Autodesk Inventor part; units mm, degrees
ref_plane "YZ Plane" through (0, 0, 0) normal (1, 0, 0) x (0, 1, 0)
ref_plane "XZ Plane" through (0, 0, 0) normal (0, 1, 0) x (-1, 0, 0)
ref_plane "XY Plane" through (0, 0, 0) normal (0, 0, 1) x (1, 0, 0)
sketch "Sketch1" plane through (0, 0, 0) normal (0, 1, 0) x (-1, 0, 0)
  line L0 (0, 0) -> (25, 0)
  line L1 (25, 0) -> (25, -28)
  line L2 (25, -28) -> (0, -28)
  line L3 (0, -28) -> (0, 0)
  dimension "d0" = 25
  dimension "d1" = 28
extrude "Extrusion1" add sketch "Sketch1" along normal blind 15
sketch "Sketch2" plane through (0, 15, 0) normal (0, 1, 0) x (1, 0, 0)
  point P0 (0, 0)
shell "Shell1" thickness 2 removed faces 1 at (-8.3333, 15, -9.3333)
sketch "Sketch3" plane through (0, 0, 0) normal (1, 0, 0) x (0, 0, -1)
  point P0 (0, 0)
sketch "Sketch4" plane through (0, 0, 0) normal (1, 0, 0) x (0, 0, -1)
  line L0 (0, 0) -> (0, 15)
  line L1 (0, 15) -> (0, 0)
  line L2 (0, 0) -> (-20, 0)
  line L3 (-20, 0) -> (-20, 2)
  arc A0 (-19, 3) -> (-20, 2) centre (-19, 2) ccw
  arc A1 (-19, 3) -> (-9.089, 9.2596) centre (-19, 13.976) ccw
  line L4 (28, 15) -> (0, 15)
  arc A2 (0, 15) -> (-9.089, 9.2596) centre (0, 4.9343) ccw
  line L5 (0, 15) -> (28, 15)
  dimension "d5" = 20
  dimension "d6" = 2
  dimension "d7" = 1
extrude "Extrusion2" add sketch "Sketch4" against normal blind 25
sketch "Sketch5" plane through (0, 0, -28) normal (0, 0, -1) x (-1, 0, 0)
  circle A0 centre (12.5, 13) radius 1.25
  line L0 (11.25, 13) -> (11.25, 15)
  line L1 (0, 15) -> (25, 15)
  line L2 (11.25, 15) -> (13.75, 15)
  line L3 (13.75, 15) -> (13.75, 13)
  point P0 (0, 0)
  dimension "d10" = 2.5
sketch "Sketch6" plane through (0, 0, -28) normal (0, 0, -1) x (-1, 0, 0)
  point P0 (0, 0)
extrude "Extrusion3" cut sketch "Sketch5" against normal up to next
sketch "Sketch7" plane through (-23, 2, -2) normal (0, 1, 0) x (1, 0, 0)
  point P0 (23, -2)
sketch "Sketch8" plane through (0, 15, 0) normal (0, 1, 0) x (1, 0, 0)
  line L0 (-2, 0) -> (-23, 0)
  line L1 (-23, 0) -> (-23, -20)
  line L2 (-23, -20) -> (-2, -20)
  line L3 (-2, -20) -> (-2, 0)
  line L4 (-12.5, 0) -> (-7.5, 0)
  line L5 (-7.5, 0) -> (-7.5, 2)
  line L6 (-7.5, 2) -> (-12.5, 2)
  line L7 (-12.5, 2) -> (-12.5, 0)
  line L8 (-12.5, 0) -> (-17.5, 0)
  line L9 (-17.5, 0) -> (-17.5, 2)
  line L10 (-17.5, 2) -> (-12.5, 2)
  line L11 (-12.5, 2) -> (-12.5, 0)
  point P0 (0, 0)
  dimension "d13" = 21
  dimension "d14" = 20
  dimension "d15" = 5
  dimension "d16" = 2
  dimension "d17" = 5
  dimension "d18" = 2
extrude "Extrusion4" cut sketch "Sketch8" against normal up to surface (13 mm away) contours L3 L2 L1 L0
extrude "Extrusion5" cut sketch "Sketch8" against normal blind 10 contours L0 L7 L6 L5 | L0 L9 L10 L7
sketch "Sketch9" plane through (-23, 2, -2) normal (0, 1, 0) x (1, 0, 0)
  line L0 (5.5, 0) -> (15.5, 0)
  line L1 (5.5, 0) -> (15.5, 0)
  line L2 (15.5, 0) -> (15.5, 10)
  line L3 (15.5, 10) -> (5.5, 10)
  line L4 (5.5, 10) -> (5.5, 0)
  point P0 (23, -2)
  dimension "d23" = 10
  dimension "d24" = 10
extrude "Extrusion6" add sketch "Sketch9" along normal up to surface (3 mm away)
properties part number "Holster"
Design review of the part built by this model. Coordinates are the model's own, in mm. A direction names the side the tool comes from. Give positions to 0.01 mm unless a question says otherwise; leave off trailing zeros. Order: outer loops, then holes, each group sorted by start corner. A loop starts at its lowest first (then second) coordinate and runs counter-clockwise, first axis right, second up. Notation, with made-up numbers: (40, 4.25) -> (76, 4.25) arc R20 ccw to (76, 35.25) -> close; hole circle Ø10 at (12.5, 56). An arc over 180 degrees is marked (long way). Write item = value, one per line. Start each with the question number.
(1) To check wall thickness, follow line 1 along X through (y, z) = (14, -13); line 2 along Z through (x, y) = (-22.25, 2.75); line 3 along X through (y, z) = (13.5, -0.5). State the ranges of each line that lie inside material, in increasing order.
(2) For pin 1 (4 mm diameter, centred on x = -9, y = 8, fed in from +Z); pin 2 (1.5 mm diameter, centred on x = -17, z = -22, fed in from +Y), all flat-tipped, find the tip position at first contact; note any pin that passes through.
(3) We need section C-C on x = -18. Write out the cut boundary in (y, z), plus the area to 3 significant figures.
(4) For faces 1 (the face through (-11.25, 14, -27)), 2 (the face through (-13, 5, -6)), 3 (the face through (-23, 8, -14)), 4 (the face through (-23.986, 13.487, 5.308)), 5 (the face through (-12, 1, 20)), list the 3-axis set-ups (+Z, -Z, +X, -X, +Y, -Y) from which the entire face can be reached by the end or side of a thin tool; tool diameter is ignored.
(5) We need section B-B on z = -7. Write out the cut boundary in (x, y), plus the area to 3 significant figures.
(6) We need section D-D on z = -23.5. Write out the cut boundary in (x, y).
(7) Mouldability with a two-part tool opening along X and no side actions: class faces 6 (the face through (-20, 8, -2)), 7 (the face through (-25, 7, -9)), 8 (the face through (0, 7, -10)) as +X half, -X half, draft (parallel to the pull), parting line (faces both ways), or undercut.
(8) We need section A-A on x = -8.25. Write out the cut boundary in (y, z), plus the area to 3 significant figures.
Numbers:
q1.line_1 = -25 to -23, -2 to 0
q1.line_2 = -28 to -26, -2 to 0
q1.line_3 = -25 to -17.5, -7.5 to 0
q2.pin_1 = 0
q2.pin_2 = 2
q3.outline = (0, -28) -> (15, -28) -> (15, -26) -> (2, -26) -> (2, -2) -> (15, -2) -> (15, 0) -> (2, 0) -> (2, 20) -> (0, 20) -> close
q3.area = 148 mm^2
q4.face_1 = +Z, -Z, +Y
q4.face_2 = +Z, +Y
q4.face_3 = +Y
q4.face_4 = +Z, +X, -X, +Y
q4.face_5 = +Z, +X, -X, +Y, -Y
q5.outline = (-25, 0) -> (0, 0) -> (0, 15) -> (-2, 15) -> (-2, 2) -> (-7.5, 2) -> (-7.5, 5) -> (-17.5, 5) -> (-17.5, 2) -> (-23, 2) -> (-23, 15) -> (-25, 15) -> close
q5.area = 132 mm^2
q6.outline = (-25, 0) -> (0, 0) -> (0, 15) -> (-2, 15) -> (-2, 2) -> (-23, 2) -> (-23, 15) -> (-25, 15) -> close
q7.face_6 = undercut
q7.face_7 = -X half
q7.face_8 = +X half
q8.outline = (0, -28) -> (15, -28) -> (15, -26) -> (2, -26) -> (2, -12) -> (5, -12) -> (5, 0) -> (2, 0) -> (2, 20) -> (0, 20) -> close
q8.area = 158 mm^2
